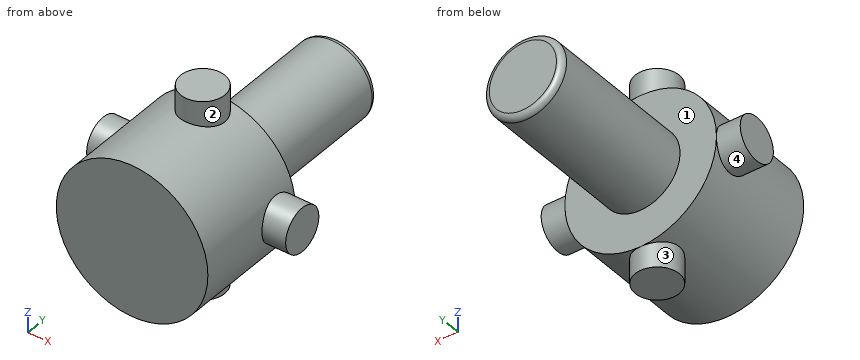
Autodesk Inventor part; units mm, degrees
ref_plane "YZ Plane" through (0, 0, 0) normal (1, 0, 0) x (0, 1, 0)
ref_plane "XZ Plane" through (0, 0, 0) normal (0, 1, 0) x (-1, 0, 0)
ref_plane "XY Plane" through (0, 0, 0) normal (0, 0, 1) x (1, 0, 0)
sketch "Esboço1" plane through (0, 0, 0) normal (0, 0, 1) x (1, 0, 0)
  line L0 (0, 0) -> (6.55, 0)
  line L1 (6.55, 0) -> (6.55, 10)
  line L2 (6.55, 10) -> (3.4, 10)
  line L3 (3.4, 10) -> (3.4, 23.5)
  line L4 (3.4, 23.5) -> (0, 23.5)
  line L5 (0, 23.5) -> (0, 0)
  dimension "d0" = 6.55
  dimension "d1" = 10
  dimension "d3" = 13.5
  dimension "d14" = 3.4
revolve "Revolução1" add sketch "Esboço1" angle 360 about axis through (0, 23.5, 0) along (0, -1, 0)
sketch "Esboço2" plane through (0, 0, 0) normal (0, 0, 1) x (1, 0, 0)
  line L0 (-6.55, 10) -> (6.55, 10)
  line L1 (0, 10) -> (0, 8.1)
  circle A0 centre (0, 8.1) radius 1.9
  point P0 (0, 0)
  dimension "d11" = 3.8
  dimension "d5" = 1.9
extrude "Extrusão1" add sketch "Esboço2" along normal mid plane 17.2
sketch "Esboço3" plane through (0, 0, 0) normal (1, 0, 0) x (0, 1, 0)
  line L0 (10, 3.4) -> (10, -3.4)
  line L1 (10, 0) -> (8.1, 0)
  circle A0 centre (8.1, 0) radius 1.9
  point P0 (0, 0)
  dimension "d8" = 1.9
extrude "Extrusão2" add sketch "Esboço3" along normal mid plane 17.2
fillet "Arredondamento2" radius 0.5 1 edges at (-3.4, 23.5, 0)
properties part number "botao_3DPrint"
Read the model definition and answer for the solid it produces. Units are mm, in the model's axes. Face numbers are marked on the shaded views. A direction names the side the tool comes from. Give positions to 0.01 mm unless a question says otherwise; leave off trailing zeros. Write each loop counter-clockwise with the first axis right and the second up, starting at its lowest first coordinate (ties: lowest second). Pieces come first, ordered by that corner, then holes. Notation, with made-up numbers: (2.25, 57) -> (16.25, 57) arc R13 cw to (16.25, 75) -> close; hole circle Ø5 at (20, -4). An arc over 180 degrees is marked (long way). Answer as a JSON object with one key per item and string values.
1) Straight lines are drawn through the part: probe 1 along Y at (x, z) = (-2.5, -3); probe 2 along Z at (x, y) = (-6.5, 8.25); probe 3 along X at (y, z) = (13.5, 0). For each, find the intervals that lie inside material, in ascending order. Write a range as from..to.
Findings below:
{"probe 1": "y = 0..10", "probe 2": "z = -1.89..1.89", "probe 3": "x = -3.4..3.4"}
2) Section C-C on x = 5.5 is taken. Write down the section's boundary in (y, z).
Findings below:
{"outline": "(0, -3.56) -> (10, -3.56) -> (10, 3.56) -> (0, 3.56) -> close"}
3) Section B-B on z = -7 is taken. Write down the section's boundary in (x, y).
Findings below:
{"outline": "circle Ø3.8 at (0, 8.1)"}
4) Flat-ended cylindrical pins translate along their axes: pin 1 Ø2 at (y, z) = (13.5, 3.5) entering from +X; pin 2 Ø6 at (x, y) = (6, 14.5) entering from +Z. Find the tip coordinate at first contact, or state that the pin passes through.
Findings below:
{"pin 1": "stops at x = 2.3", "pin 2": "stops at z = 1.6"}
5) A tool of negligible diameter and unlimited length cuts with its end or side. For the marked faces 1, 2, 3 and 4, from which of +Z, -Z, +X, -X, +Y, -Y can it reach the whole face along a straight path? Write none if from no direction.
Findings below:
{"face 1": "+Y", "face 2": "+Z", "face 3": "-Z", "face 4": "-X"}
6) Section A-A on y = 8.1 is taken. Write down the section's boundary in (x, z).
Findings below:
{"outline": "(-8.6, -1.9) -> (-6.27, -1.9) arc R6.55 ccw to (-1.9, -6.27) -> (-1.9, -8.6) -> (1.9, -8.6) -> (1.9, -6.27) arc R6.55 ccw to (6.27, -1.9) -> (8.6, -1.9) -> (8.6, 1.9) -> (6.27, 1.9) arc R6.55 ccw to (1.9, 6.27) -> (1.9, 8.6) -> (-1.9, 8.6) -> (-1.9, 6.27) arc R6.55 ccw to (-6.27, 1.9) -> (-8.6, 1.9) -> close"}
7) Section D-D on y = 18.5 is taken. Write down the section's boundary in (x, z).
Findings below:
{"outline": "circle Ø6.8 at (0, 0)"}
